```python
from build123d import *

# Parameters (mm, degrees)
ESBO_O1_W                = 160
ESBO_O1_H                = 12.75
ESBO_O1_R                = 1.7
RESSALTO_EXTRUS_O1_DEPTH = 2
ESBO_O2_R                = 3
RESSALTO_EXTRUS_O2_DEPTH = 5


with BuildPart() as part:
    # Esboço1 → Ressalto-extrusão1 (new body)
    with BuildSketch(Plane(origin=(0, 0, 0), x_dir=(0, 0, -1), z_dir=(1, 0, 0))):
        Rectangle(ESBO_O1_W, ESBO_O1_H)
        with Locations((-74, 0.175)):
            Circle(ESBO_O1_R, mode=Mode.SUBTRACT)
        with Locations((-26, 0.175)):
            Circle(ESBO_O1_R, mode=Mode.SUBTRACT)
        with Locations((26, 0.175)):
            Circle(ESBO_O1_R, mode=Mode.SUBTRACT)
        with Locations((74, 0.175)):
            Circle(ESBO_O1_R, mode=Mode.SUBTRACT)
    extrude(amount=RESSALTO_EXTRUS_O1_DEPTH)

    # Esboço2 → Ressalto-extrusão2 (add)
    with BuildSketch(Plane(origin=(2, 0, 0), x_dir=(0, 0, -1), z_dir=(1, 0, 0))):
        with Locations((0.17, -0.555)):
            Circle(ESBO_O2_R)
        with Locations((50.77, -0.555)):
            Circle(ESBO_O2_R)
        with Locations((-50.53, -0.555)):
            Circle(ESBO_O2_R)
    extrude(amount=RESSALTO_EXTRUS_O2_DEPTH)


solid = part.part
```
Read the model definition and answer for the solid it produces. Units are mm, in the model's axes. A direction names the side the tool comes from. Coordinates: 2 decimals unless noted, no trailing zeros. Loops run counter-clockwise (first coordinate to the right, second up) from the corner with the lowest first, then second, coordinate; pieces in that order, holes last. Notation, with made-up numbers: (63.25, 66) -> (72.25, 66) arc R26 cw to (72.25, 94) -> close; hole circle Ø4 at (87.5, 40.25). An arc over 180 degrees is marked (long way). Return JSON: item names as keys, results as strings.
Item 1: Find the intervals of material crossed by probe 1 along Z at (x, y) = (6.5, -0.75); probe 2 along Z at (x, y) = (3.25, 1.5); probe 3 along Y at (x, z) = (1.3, 74) (3 decimals), in increasing order.
Answers:
{"probe 1": "z = -53.76 to -47.78, -3.16 to 2.82, 47.54 to 53.52", "probe 2": "z = -52.96 to -48.58, -2.36 to 2.02, 48.34 to 52.72", "probe 3": "y = -6.375 to -1.525, 1.875 to 6.375"}
Item 2: For a pull along Y with two mould halves and no side action, classify faces 3 (the cylindrical face through (1, 0.2, 75.7)), 4 (the cylindrical face through (1, 0.2, -72.3)), 5 (the cylindrical face through (4.46, -2.38, 2.21)), 6 (the flat face through (7, -1, 51)) as +Y half, -Y half, draft (parallel to the pull), parting line (faces both ways), or undercut.
Answers:
{"face 3": "undercut", "face 4": "undercut", "face 5": "parting line", "face 6": "draft"}
Item 3: Find section A-A (z = -74). Determine the outline of the cut face in (x, y) (3 decimals).
Answers:
{"outline": "(0, -6.375) -> (2, -6.375) -> (2, -1.525) -> (0, -1.525) -> close; (0, 1.875) -> (2, 1.875) -> (2, 6.375) -> (0, 6.375) -> close"}
Item 4: Find section B-B (z = -0.17). Determine the outline of the cut face in (x, y) (3 decimals).
Answers:
{"outline": "(0, -6.375) -> (2, -6.375) -> (2, -3.555) -> (7, -3.555) -> (7, 2.445) -> (2, 2.445) -> (2, 6.375) -> (0, 6.375) -> close"}
Item 5: Find section C-C (y = 4). Determine the outline of the cut face in (x, z).
Answers:
{"outline": "(0, -80) -> (2, -80) -> (2, 80) -> (0, 80) -> close"}
Item 6: Find section D-D (x = 5.5). Determine the outline of the cut face in (y, z) (3 decimals).
Answers:
{"outline": "circle Ø6 at (-0.555, -50.77); circle Ø6 at (-0.555, -0.17); circle Ø6 at (-0.555, 50.53)"}
Item 7: For faces 1 (the cylindrical face through (4.46, 0.35, 47.67)), 2 (the cylindrical face through (0.99, -0.48, -27.57)), determine the directions among +Z, -Z, +X, -X, +Y, -Y from which every point of the face is accessible in a straight line to the end or side of a thin tool.
Answers:
{"face 1": "+X", "face 2": "+X, -X"}
Item 8: Flat-ended cylindrical pins translate along their axes: P1, Ø3, axis at x = 5.5, y = -4.5, coming from the +Z side; P2, Ø1, axis at x = 3, z = -15, coming from the +Y side; P3, Ø5.5, axis at y = 0.175, z = 74, coming from the +X side; P4, Ø1.5, axis at x = 3, y = -0.5, coming from the +Z side. Find the tip coordinate at first contact, or state that the pin passes through.
Answers:
{"P1": "stops at z = 52.27", "P2": "passes through", "P3": "stops at x = 2", "P4": "stops at z = 53.53"}
